from build123d import *

# Parameters (mm, degrees)
SKETCH1_W           = 72.2
SKETCH1_H           = 88.4
BOSS_EXTRUDE1_DEPTH = 40
CUT_EXTRUDE4_DEPTH  = 69
FILLET1_R           = 10
SKETCH3_R           = 0.9
CUT_EXTRUDE5_DEPTH  = 20


with BuildPart() as part:
    # Sketch1 → Boss-Extrude1 (new body)
    with BuildSketch(Plane(origin=(0, 0, 0), x_dir=(1, 0, 0), z_dir=(0, 1, 0))):
        with Locations((36.1, 44.2)):
            Rectangle(SKETCH1_W, SKETCH1_H)
    extrude(amount=BOSS_EXTRUDE1_DEPTH)

    # Sketch2 → Cut-Extrude4 (cut)
    with BuildSketch(Plane(origin=(72.2, 0, 0), x_dir=(0, 0, -1), z_dir=(1, 0, 0))):
        Polygon((3.2, 12.8), (3.2, 3.2), (85.2, 3.2), (85.2, 12.8), (79.2, 12.8), (79.2, 14.8), (85.2, 14.8), (85.2, 16.8), (79.2, 16.8), (79.2, 36.8), (44.2, 36.8), (9.2, 36.8), (9.2, 16.8), (3.2, 16.8), (3.2, 14.8), (9.2, 14.8), (9.2, 12.8), align=None)
    extrude(amount=-CUT_EXTRUDE4_DEPTH, mode=Mode.SUBTRACT)

    # Fillet1
    fillet1_edges = [part.edges().sort_by_distance(p)[0] for p in [
        (36.1, 40, -88.4),
        (0, 40, -44.2),
        (0, 20, -88.4),
        (0, 20, 0),
        (36.1, 40, 0),
    ]]
    fillet(fillet1_edges, radius=FILLET1_R)

    # Sketch3 → Cut-Extrude5 (cut)
    with BuildSketch(Plane(origin=(72.2, 0, 0), x_dir=(0, 0, -1), z_dir=(1, 0, 0))):
        with Locations((4.6, 23)):
            Circle(SKETCH3_R)
        with Locations((83.8, 23)):
            Circle(SKETCH3_R)
    extrude(amount=-CUT_EXTRUDE5_DEPTH, mode=Mode.SUBTRACT)


solid = part.part
CAD build for the part. Positions are in the model's coordinates, mm. A direction names the side the tool comes from. Round coordinates to 2 decimals unless told otherwise and drop trailing zeros. Write each loop counter-clockwise with the first axis right and the second up, starting at its lowest first coordinate (ties: lowest second). Pieces come first, ordered by that corner, then holes. Notation, with made-up numbers: M 13.25,-6 L 18.25,-6 A25 cw 18.25,10 Z; hole C -28.75,59.25 d2. An arc over 180 degrees is marked long. Use a Markdown table: item, result. Add a question column.
1. Slice it at C-C on y = 29. Give the cut face in (x, z).
2. Drill centre lines: probe 1 along Z at (x, y) = (68, 29.5); probe 2 along Y at (x, z) = (54, -71.5); probe 3 along Z at (x, y) = (66.5, 11). Where is each one in solid material? Low to high.
3. Slice it at A-A on x = 63.5. Give the cut face in (y, z), then the cut area to 3 significant figures.
4. Pull direction Z, two halves, no side cores. Call faces 1 (the face through (41, 40, -45)), 2 (the face through (38, 8, -85.2)), 3 (the face through (41.54, 36.99, -85.55)): released by +Z, released by -Z, zero draft, split by the parting line, or undercut.
5. 3-axis set-ups, long thin cutter, end or side, ignore diameter. For faces 4 (the face through (72.2, 2, -44)), 5 (the face through (38, 12.8, -82)): which of +Z, -Z, +X, -X, +Y, -Y reach the whole face in a straight line?
6. Slice it at D-D on x = 9. Give the cut face in (y, z), then the cut area to 3 significant figures.
7. Slice it at B-B on z = -18. Give the cut face in (x, y).
8. Flat gauge pins, fed straight in: P1, Ø2, axis at x = 36.5, y = 35.5, coming from the +Z side; P2, Ø6.5, axis at x = 54.5, z = -6, coming from the +Y side; P3, Ø17, axis at y = 26, z = -63.5, coming from the +X side. Where does each tip first touch, or does it go through?
Reply:
| question | item | result |
|---|---|---|
| 1 | outline | M 0,-78.4 A10 ccw 10,-88.4 L 72.2,-88.4 L 72.2,-79.2 L 3.2,-79.2 L 3.2,-9.2 L 72.2,-9.2 L 72.2,0 L 10,0 A10 ccw 0,-10 Z |
| 2 | probe 1 | z = -88.4 to -79.2, -9.2 to 0 |
| 2 | probe 2 | y = 0 to 3.2, 36.8 to 40 |
| 2 | probe 3 | z = -88.4 to -85.2, -3.2 to 0 |
| 3 | outline | M 0,-88.4 L 30,-88.4 A10 ccw 40,-78.4 L 40,-10 A10 ccw 30,0 L 0,0 Z; hole M 3.2,-85.2 L 12.8,-85.2 L 12.8,-79.2 L 14.8,-79.2 L 14.8,-85.2 L 16.8,-85.2 L 16.8,-79.2 L 36.8,-79.2 L 36.8,-9.2 L 16.8,-9.2 L 16.8,-3.2 L 14.8,-3.2 L 14.8,-9.2 L 12.8,-9.2 L 12.8,-3.2 L 3.2,-3.2 Z; hole C 23,-83.8 d1.8; hole C 23,-4.6 d1.8 |
| 3 | area | 997 mm^2 |
| 4 | face 1 | zero draft |
| 4 | face 2 | undercut |
| 4 | face 3 | released by -Z |
| 5 | face 4 | +Z, -Z, +X, +Y, -Y |
| 5 | face 5 | +X |
| 6 | outline | M 0,-88.35 L 30,-88.35 A9.95 ccw 39.95,-78.4 L 39.95,-10 A9.95 ccw 30,-0.05 L 0,-0.05 Z; hole M 3.2,-85.2 L 12.8,-85.2 L 12.8,-79.2 L 14.8,-79.2 L 14.8,-85.2 L 16.8,-85.2 L 16.8,-79.2 L 36.8,-79.2 L 36.8,-9.2 L 16.8,-9.2 L 16.8,-3.2 L 14.8,-3.2 L 14.8,-9.2 L 12.8,-9.2 L 12.8,-3.2 L 3.2,-3.2 Z |
| 6 | area | 994 mm^2 |
| 7 | outline | M 0,0 L 72.2,0 L 72.2,3.2 L 3.2,3.2 L 3.2,36.8 L 72.2,36.8 L 72.2,40 L 10,40 A10 ccw 0,30 Z |
| 8 | P1 | stops at z = -1.07 |
| 8 | P2 | stops at y = 39.97 |
| 8 | P3 | stops at x = 3.2 |
